Autodesk Inventor part; units mm, degrees
ref_plane "YZ Plane" through (0, 0, 0) normal (1, 0, 0) x (0, 1, 0)
ref_plane "XZ Plane" through (0, 0, 0) normal (0, 1, 0) x (-1, 0, 0)
ref_plane "XY Plane" through (0, 0, 0) normal (0, 0, 1) x (1, 0, 0)
sketch "スケッチ1" plane through (0, 0, 0) normal (0, 0, 1) x (1, 0, 0)
  point P0 (0, 0)
sketch "スケッチ2" plane through (0, 0, 0) normal (0, 0, 1) x (1, 0, 0)
  line L0 (-16, 16) -> (16, 16)
  line L1 (16, 16) -> (16, -16)
  line L2 (16, -16) -> (-16, -16)
  line L3 (-16, -16) -> (-16, 16)
  line L4 (-16, 16) -> (16, -16) construction
  line L5 (16, 16) -> (-16, -16) construction
  line L6 (-15.2, 15.2) -> (15.2, 15.2)
  line L7 (15.2, 15.2) -> (15.2, -15.2)
  line L8 (15.2, -15.2) -> (-15.2, -15.2)
  line L9 (-15.2, -15.2) -> (-15.2, 15.2)
  line L10 (-15.2, 15.2) -> (15.2, -15.2) construction
  line L11 (15.2, 15.2) -> (-15.2, -15.2) construction
  point P0 (0, 0)
  point P1 (0, 0)
  dimension "d0" = 32
  dimension "d1" = 32
  dimension "d2" = 30.4
  dimension "d3" = 30.4
extrude "押し出し1" add sketch "スケッチ2" along normal blind 224.0259
sketch "スケッチ3" plane through (-16, 16, 0) normal (0, 1, 0) x (1, 0, 0)
  line L0 (32, -224.0259) -> (0, -224.0259)
  point P0 (16, 0)
  point P1 (16, -208.0259)
  dimension "d6" = 16
hole "穴1" at (0, 16, 208.0259) direction (0, -1, 0) diameter 10 end through all
sketch "スケッチ4" plane through (-16, 16, 0) normal (0, 1, 0) x (1, 0, 0)
  point P0 (16, 0)
sketch "スケッチ5" plane through (-16, 16, 0) normal (0, 1, 0) x (1, 0, 0)
  line L0 (0, 0) -> (32, -12.9008)
  line L1 (32, 0) -> (32, -224.0259)
  line L2 (0, 0) -> (34.5026, 0) construction
  line L3 (32, -12.9008) -> (32, 0)
  line L4 (0, 0) -> (32, 0)
  line L5 (32, 0) -> (0, 0)
  point P0 (16, 0)
  dimension "d14" = 21.957
extrude "押し出し2" cut sketch "スケッチ5" against normal blind 32
properties part number "アッカーマンpipe1"
Source: CAD feature listing. Evaluate the final solid. Frame: model axes, mm. A direction names the side the tool comes from. Give positions to 0.01 mm unless a question says otherwise; leave off trailing zeros. Loops run counter-clockwise (first coordinate to the right, second up) from the corner with the lowest first, then second, coordinate; pieces in that order, holes last. Notation, with made-up numbers: (20, 17.5) -> (57, 17.5) arc R23 ccw to (57, 30.5) -> close; hole circle Ø8 at (-38.75, 75.25). An arc over 180 degrees is marked (long way). Use a Markdown table: item, result. Add a question column.
1) Section query D-D, the plane x = 13. Return the cut outline in (y, z), then the cut area to 3 significant figures.
2) First-contact query: pin 1 (6 mm diameter, centred on x = 0, z = 208.03, fed in from +Y). Flat tip, straight axial feed; report the tip coordinate or a pass-through.
3) Reachability of faces 5 (the face through (16, 0, 117)), 6 (the face through (15.2, 0, 117)) from +Z, -Z, +X, -X, +Y, -Y: full face, straight path, thin tool, end or side. Return the list, or none.
4) Section query C-C, the plane x = 2.5. Return the cut outline in (y, z), then the cut area to 3 significant figures.
5) Section query A-A, the plane y = -8. Return the cut outline in (x, z), then the cut area to 3 significant figures.
6) Line query: line 1 along Y through (x, z) = (-4.5, 11); line 2 along Z through (x, y) = (0, 15.6). Output: solid intervals per line, ascending. Write a range as [from, to].
7) Pull-direction query (Z, two-part tool) for faces 1 (the face through (-1.502, 15.594, 212.795)), 2 (the face through (-1.502, -15.606, 212.795)), 3 (the face through (-15.5, 0.1, 224.026)), 4 (the face through (0, 15.2, 111)); classes: +Z half, -Z half, draft (parallel to the pull), parting line (faces both ways), or undercut.
8) Section query B-B, the plane z = 173. Return the cut outline in (x, y).
Numbers:
| question | item | result |
|---|---|---|
| 1 | outline | (-16, 11.69) -> (-15.2, 11.69) -> (-15.2, 224.03) -> (-16, 224.03) -> close; (15.2, 11.69) -> (16, 11.69) -> (16, 224.03) -> (15.2, 224.03) -> close |
| 1 | area | 340 mm2 |
| 2 | pin 1 | passes through |
| 3 | face 5 | +Z, -Z, +X, +Y, -Y |
| 3 | face 6 | +Z, -Z |
| 4 | outline | (-16, 7.46) -> (-15.2, 7.46) -> (-15.2, 203.7) -> (-16, 203.7) -> close; (-16, 212.36) -> (-15.2, 212.36) -> (-15.2, 224.03) -> (-16, 224.03) -> close; (15.2, 7.46) -> (16, 7.46) -> (16, 203.7) -> (15.2, 203.7) -> close; (15.2, 212.36) -> (16, 212.36) -> (16, 224.03) -> (15.2, 224.03) -> close |
| 4 | area | 333 mm2 |
| 5 | outline | (-16, 0) -> (-15.2, 0.32) -> (-15.2, 224.03) -> (-16, 224.03) -> close; (15.2, 12.58) -> (16, 12.9) -> (16, 224.03) -> (15.2, 224.03) -> close |
| 5 | area | 348 mm2 |
| 6 | line 1 | y = [-16, -15.2], [15.2, 16] |
| 6 | line 2 | z = [6.45, 203.03], [213.03, 224.03] |
| 7 | face 1 | undercut |
| 7 | face 2 | undercut |
| 7 | face 3 | +Z half |
| 7 | face 4 | draft |
| 8 | outline | (-16, -16) -> (16, -16) -> (16, 16) -> (-16, 16) -> close; hole (-15.2, -15.2) -> (15.2, -15.2) -> (15.2, 15.2) -> (-15.2, 15.2) -> close |
